The listing builds one solid part. Answer for the finished solid, in the listing's coordinates (mm). A direction names the side the tool comes from. Round coordinates to 2 decimals unless told otherwise and drop trailing zeros. Write each loop counter-clockwise with the first axis right and the second up, starting at its lowest first coordinate (ties: lowest second). Pieces come first, ordered by that corner, then holes. Notation, with made-up numbers: (-19, -26.75) - (19, -26.75) arc R33 cw to (19, 11.25) - close; hole circle Ø7 at (72, -33.75). An arc over 180 degrees is marked (long way). Answer in a Markdown table with one row per item.
from build123d import *

# Parameters (mm, degrees)
SKIZZE1_R                       = 11.25
SKIZZE1_R_2                     = 5.25
AUFSATZ_LINEAR_AUSTRAGEN1_DEPTH = 10
AUFSATZ_LINEAR_START            = 6
SKIZZE2_W                       = 10
SKIZZE2_H                       = 10
AUFSATZ_LINEAR_AUSTRAGEN2_DEPTH = 11.4
SKIZZE3_R                       = 2.45
SCHNITT_LINEAR_AUSTRAGEN1_DEPTH = 10
SKIZZE4_R                       = 1.45
SCHNITT_LINEAR_AUSTRAGEN2_DEPTH = 8
VERRUNDUNG2_R                   = 5
VERRUNDUNG1_R                   = 1
FASE1_SIZE                      = 0.5


with BuildPart() as part:
    # Skizze1 → Aufsatz-Linear austragen1 (new body)
    with BuildSketch(Plane.XY):
        Circle(SKIZZE1_R)
        Circle(SKIZZE1_R_2, mode=Mode.SUBTRACT)
    extrude(amount=AUFSATZ_LINEAR_AUSTRAGEN1_DEPTH)

    # Skizze2 → Aufsatz-Linear austragen2 (add)
    with BuildSketch(Plane(origin=(0, 0, 0), x_dir=(1, 0, 0), z_dir=(0, 1, 0)).offset(AUFSATZ_LINEAR_START)):
        with Locations((0, -5)):
            Rectangle(SKIZZE2_W, SKIZZE2_H)
    aufsatz_linear_austragen2 = extrude(amount=AUFSATZ_LINEAR_AUSTRAGEN2_DEPTH)

    # Skizze3 → Schnitt-Linear austragen1 (cut)
    with BuildSketch(Plane(origin=(0, 17.4, 0), x_dir=(1, 0, 0), z_dir=(0, 1, 0))):
        with Locations(Location((0, -5, 0), (0, 0, 270))):
            Circle(SKIZZE3_R)
    schnitt_linear_austragen1 = extrude(amount=-SCHNITT_LINEAR_AUSTRAGEN1_DEPTH, mode=Mode.SUBTRACT)

    # Spiegeln1: Aufsatz-Linear austragen2, Schnitt-Linear austragen1 across plane
    add(aufsatz_linear_austragen2.mirror(Plane.ZX))
    add(schnitt_linear_austragen1.mirror(Plane.ZX), mode=Mode.SUBTRACT)

    # Skizze4 → Schnitt-Linear austragen2 (cut)
    with BuildSketch(Plane.XY.offset(10)):
        with Locations((8, 0)):
            Circle(SKIZZE4_R)
        with Locations(Location((-8, 0, 0), (0, 0, 180))):
            Circle(SKIZZE4_R)
    extrude(amount=-SCHNITT_LINEAR_AUSTRAGEN2_DEPTH, mode=Mode.SUBTRACT)

    # Verrundung2
    verrundung2_edges = [part.edges().sort_by_distance(p)[0] for p in [
        (-5, 10.077822185, 5),
        (5, 10.077822185, 5),
        (5, -10.077822185, 5),
        (-5, -10.077822185, 5),
    ]]
    fillet(verrundung2_edges, radius=VERRUNDUNG2_R)

    # Verrundung1
    verrundung1_edges = [part.edges().sort_by_distance(p)[0] for p in [
        (5, 17.4, 5),
        (-5, 17.4, 5),
        (5, -17.4, 5),
        (-5, -17.4, 5),
    ]]
    fillet(verrundung1_edges, radius=VERRUNDUNG1_R)

    # Fase1
    fase1_edges = [part.edges().sort_by_distance(p)[0] for p in [
        (-5, 14.604344229, 10),
        (-5, -14.604344229, 10),
        (0, -17.4, 10),
        (5, -14.604344229, 10),
        (5, 14.604344229, 10),
        (-4.707106781, -17.107106781, 10),
        (4.707106781, -17.107106781, 10),
        (4.707106781, 17.107106781, 10),
        (-4.707106781, 17.107106781, 10),
        (-5, 14.604344229, 0),
        (5, -14.604344229, 0),
        (0, -17.4, 0),
        (-5, -14.604344229, 0),
        (5, 14.604344229, 0),
        (-4.707106781, -17.107106781, 0),
        (4.707106781, -17.107106781, 0),
        (4.707106781, 17.107106781, 0),
        (-4.707106781, 17.107106781, 0),
        (-5.25, 0, 0),
        (-5.25, 0, 10),
        (6.55, 0, 10),
        (-6.55, 0, 10),
        (-11.25, 0, 0),
        (-11.25, 0, 10),
        (11.25, 0, 10),
        (11.25, 0, 0),
        (-5.506414829, -10.616043409, 10),
        (-5.506414829, -10.616043409, 0),
        (-5.506414829, 10.616043409, 10),
        (-5.506414829, 10.616043409, 0),
        (5.506414829, 10.616043409, 0),
        (5.506414829, 10.616043409, 10),
        (5.506414829, -10.616043409, 0),
        (5.506414829, -10.616043409, 10),
        (0, 17.4, 0),
        (0, 17.4, 10),
    ]]
    chamfer(fase1_edges, length=FASE1_SIZE)


solid = part.part
(1) For a pull along Z with two mould halves and no side action, classify faces 1 (the flat face through (5, 4, 10)), 2 (the flat face through (0, 7.4, 5)), 3 (the cylindrical face through (-11.25, 0.14, 4.94)) as pulls with the +Z half, pulls with the -Z half, needs draft (parallel to the pull), parting line crosses it, or undercut.
Checked values:
| item | result |
|---|---|
| face 1 | pulls with the +Z half |
| face 2 | undercut |
| face 3 | needs draft |
(2) Section A-A (x = 0) is taken. Give the vertices of the cut face in (y, z).
Checked values:
| item | result |
|---|---|
| outline | (-17.4, 0.5) - (-16.9, 0) - (-5.75, 0) - (-5.25, 0.5) - (-5.25, 9.5) - (-5.75, 10) - (-16.9, 10) - (-17.4, 9.5) - (-17.4, 7.45) - (-7.4, 7.45) - (-7.4, 2.55) - (-17.4, 2.55) - close; (5.25, 0.5) - (5.75, 0) - (16.9, 0) - (17.4, 0.5) - (17.4, 2.55) - (7.4, 2.55) - (7.4, 7.45) - (17.4, 7.45) - (17.4, 9.5) - (16.9, 10) - (5.75, 10) - (5.25, 9.5) - close |
(3) Section D-D (z = 5) is taken. Give the vertices of the cut face in (x, y), and give its area (3 significant figures).
Checked values:
| item | result |
|---|---|
| outline | (-6.92, -8.87) arc R5 cw to (-5, -12.81) - (-5, -16.4) arc R1 ccw to (-4, -17.4) - (-2.45, -17.4) - (-2.45, -7.4) - (2.45, -7.4) - (2.45, -17.4) - (4, -17.4) arc R1 ccw to (5, -16.4) - (5, -12.81) arc R5 cw to (6.92, -8.87) arc R11.25 ccw to (6.92, 8.87) arc R5 cw to (5, 12.81) - (5, 16.4) arc R1 ccw to (4, 17.4) - (2.45, 17.4) - (2.45, 7.4) - (-2.45, 7.4) - (-2.45, 17.4) - (-4, 17.4) arc R1 ccw to (-5, 16.4) - (-5, 12.81) arc R5 cw to (-6.92, 8.87) arc R11.25 ccw to start; hole circle Ø2.9 at (-8, 0); hole circle Ø10.5 at (0, 0); hole circle Ø2.9 at (8, 0) |
| area | 334 mm2 |
(4) Section C-C (y = 0) is taken. Give the vertices of the cut face in (x, z).
Checked values:
| item | result |
|---|---|
| outline | (-11.25, 0.5) - (-10.75, 0) - (-5.75, 0) - (-5.25, 0.5) - (-5.25, 9.5) - (-5.75, 10) - (-6.05, 10) - (-6.55, 9.5) - (-6.55, 2) - (-9.45, 2) - (-9.45, 9.5) - (-9.95, 10) - (-10.75, 10) - (-11.25, 9.5) - close; (5.25, 0.5) - (5.75, 0) - (10.75, 0) - (11.25, 0.5) - (11.25, 9.5) - (10.75, 10) - (9.95, 10) - (9.45, 9.5) - (9.45, 2) - (6.55, 2) - (6.55, 9.5) - (6.05, 10) - (5.75, 10) - (5.25, 9.5) - close |
(5) For faces 4 (the flat face through (5, 15, 5)), 5 (the flat face through (-5, 15, 5)), 6 (the cylindrical face through (-0.938, -12.47, 7.263)), determine the directions among +Z, -Z, +X, -X, +Y, -Y from which every point of the face is accessible in a straight line to the end or side of a thin tool.
Checked values:
| item | result |
|---|---|
| face 4 | +Z, -Z, +X, +Y |
| face 5 | +Z, -Z, -X, +Y |
| face 6 | -Y |
(6) Find the intervals of material crossed by line 1 (X direction, y = 14.5, z = 5); line 2 (Y direction, x = 4.5, z = 1.75); line 3 (X direction, y = 12, z = 5), in increasing order.
Checked values:
| item | result |
|---|---|
| line 1 | x = -5 to -2.45, 2.45 to 5 |
| line 2 | y = -17.27 to -2.7, 2.7 to 17.27 |
| line 3 | x = -5.07 to -2.45, 2.45 to 5.07 |
(7) Section B-B (y = 13.5) is taken. Give the vertices of the cut face in (x, z).
Checked values:
| item | result |
|---|---|
| outline | (-5, 0.5) - (-4.5, 0) - (4.5, 0) - (5, 0.5) - (5, 9.5) - (4.5, 10) - (-4.5, 10) - (-5, 9.5) - close; hole circle Ø4.9 at (0, 5) |
(8) Flat-ended cylindrical pins translate along their axes: pin 1 (6 mm diameter, centred on y = 12, z = 3, fed in from -X); pin 2 (0.9 mm diameter, centred on x = 7.5, y = -0.5, fed in from +Z); pin 3 (4 mm diameter, centred on x = 0, z = 5, fed in from +Y). Find the tip coordinate at first contact, or state that the pin passes through.
Checked values:
| item | result |
|---|---|
| pin 1 | stops at x = -6.76 |
| pin 2 | stops at z = 2 |
| pin 3 | stops at y = 7.4 |
